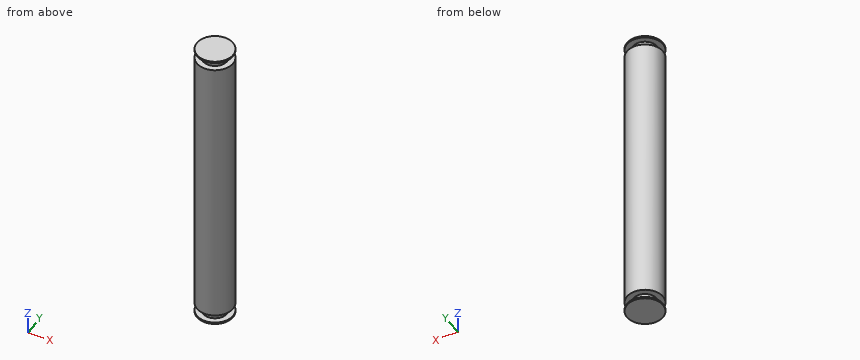
```python
from build123d import *

# Parameters (mm, degrees)
SKETCH1_R           = 22.5
BOSS_EXTRUDE1_DEPTH = 173.335
SKETCH2_R           = 15
BOSS_EXTRUDE2_DEPTH = 10
BOSS_EXTRUDE3_START = 2
SKETCH3_R           = 22.5
BOSS_EXTRUDE3_DEPTH = 2


with BuildPart() as part:
    # Sketch1 → Boss-Extrude1 (new, symmetric)
    with BuildSketch(Plane.XY):
        Circle(SKETCH1_R)
    extrude(amount=BOSS_EXTRUDE1_DEPTH, both=True)

    # Sketch2 → Boss-Extrude2 (add)
    with BuildSketch(Plane.XY.offset(173.335)):
        Circle(SKETCH2_R)
    boss_extrude2 = extrude(amount=BOSS_EXTRUDE2_DEPTH)

    # Sketch3 → Boss-Extrude3 (add)
    with BuildSketch(Plane.XY.offset(183.335).offset(BOSS_EXTRUDE3_START)):
        Circle(SKETCH3_R)
    boss_extrude3 = extrude(amount=-BOSS_EXTRUDE3_DEPTH)

    # Mirror1: Boss-Extrude2, Boss-Extrude3 across plane
    add(boss_extrude2.mirror(Plane.XY))
    add(boss_extrude3.mirror(Plane.XY))


solid = part.part
```
Part model, mm, in its own coordinate system. Round coordinates to 2 decimals unless told otherwise and drop trailing zeros. Write each loop counter-clockwise with the first axis right and the second up, starting at its lowest first coordinate (ties: lowest second). Pieces come first, ordered by that corner, then holes. Notation, with made-up numbers: (-33.75, 35.25) -> (-7.75, 35.25) arc R27 cw to (-7.75, 74.25) -> close; hole circle Ø1 at (32.25, -33). An arc over 180 degrees is marked (long way). Return JSON: item names as keys, results as strings. Group by question number.
Q1. Saw through at C-C on z = 95. Write the cut outline in (x, y).
Q2. Probe L1, parallel to Z at x = -15, y = -10.5 (3 decimals); L2, parallel to X at y = -1, z = -43. List the from-to ranges inside material, lowest first. Write a range as [from, to].
Q3. Saw through at A-A on y = 0. Write the cut outline in (x, z) (3 decimals).
Q4. Pin check, flat tips, straight feed: pin 1 (2 mm diameter, centred on x = -15, z = -19, fed in from -Y); pin 2 (3 mm diameter, centred on y = 9.5, z = -87.5, fed in from -X); pin 3 (10 mm diameter, centred on y = -7.5, z = -10, fed in from +X). Stop position of each tip, or through.
Answer:
{
 "1": {"outline": "circle Ø45 at (0, 0)"},
 "2": {"L1": "[-185.335, -183.335], [-173.335, 173.335], [183.335, 185.335]", "L2": "[-22.48, 22.48]"},
 "3": {"outline": "(-22.5, -185.335) -> (22.5, -185.335) -> (22.5, -183.335) -> (15, -183.335) -> (15, -173.335) -> (22.5, -173.335) -> (22.5, 173.335) -> (15, 173.335) -> (15, 183.335) -> (22.5, 183.335) -> (22.5, 185.335) -> (-22.5, 185.335) -> (-22.5, 183.335) -> (-15, 183.335) -> (-15, 173.335) -> (-22.5, 173.335) -> (-22.5, -173.335) -> (-15, -173.335) -> (-15, -183.335) -> (-22.5, -183.335) -> close"},
 "4": {"pin 1": "y = -17.61", "pin 2": "x = -21.03", "pin 3": "x = 22.36"}
}
